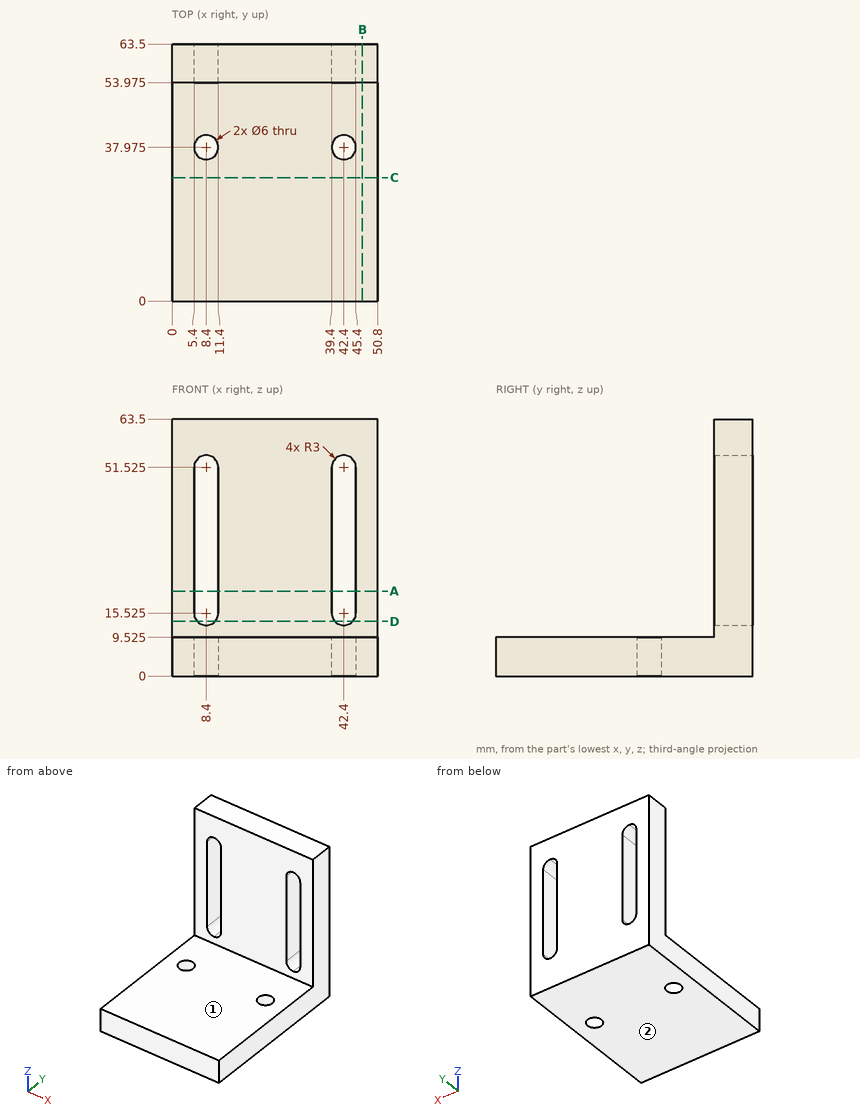
For this review, use the dimensioned drawing (mm, ordinates from the lowest corner) and the shaded views. A direction names the side the tool comes from. Give positions to 0.01 mm unless a question says otherwise; leave off trailing zeros. Write each loop counter-clockwise with the first axis right and the second up, starting at its lowest first coordinate (ties: lowest second). Pieces come first, ordered by that corner, then holes. Notation, with made-up numbers: M 7,-13 L 38,-13 A20 ccw 38,3 Z; hole C 61.25,77.25 d8. An arc over 180 degrees is marked long. Answer as a JSON object with one key per item and string values. Group by question number.
Item 1: For probe 1 along Y at (x, z) = (42.4, 6.25) (3 decimals); probe 2 along Z at (x, y) = (17, 18.5) (3 decimals); probe 3 along X at (y, z) = (55, 52), list the stretches that pass through material, from the lowest coordinate up. Write a range as [from, to].
Item 2: For pin 1 Ø9.5 at (x, y) = (8.4, 37.975) entering from +Z (3 decimals); pin 2 Ø4 at (x, y) = (28.5, 33) entering from -Z; pin 3 Ø12 at (x, z) = (43.5, 53) entering from -Y (3 decimals); pin 4 Ø12 at (y, z) = (45.5, 22.5) entering from -X, all flat-tipped, find the tip position at first contact; note any pin that passes through.
Item 3: Consider section B-B on x = 47. Write out the cut boundary in (y, z) (3 decimals).
Item 4: Consider section D-D on z = 13.5. Write out the cut boundary in (x, y) (3 decimals).
Item 5: Consider section A-A on z = 21. Write out the cut boundary in (x, y) (3 decimals).
Item 6: Tool access review of the marked faces 1 and 2: name each direction out of +Z, -Z, +X, -X, +Y, -Y from which nothing blocks a thin tool from reaching the whole face with its end or side.
Item 7: Consider section C-C on y = 30.5. Write out the cut boundary in (x, z) (3 decimals), plus the area to 3 significant figures.
Check result:
{
 "1": {"probe 1": "y = [0, 34.975], [40.975, 63.5]", "probe 2": "z = [0, 9.525]", "probe 3": "x = [0, 5.44], [11.36, 39.44], [45.36, 50.8]"},
 "2": {"pin 1": "stops at z = 9.525", "pin 2": "stops at z = 0", "pin 3": "stops at y = 53.975", "pin 4": "passes through"},
 "3": {"outline": "M 0,0 L 63.5,0 L 63.5,63.5 L 53.975,63.5 L 53.975,9.525 L 0,9.525 Z"},
 "4": {"outline": "M 0,53.975 L 6.187,53.975 L 6.187,63.5 L 0,63.5 Z; M 10.613,53.975 L 40.187,53.975 L 40.187,63.5 L 10.613,63.5 Z; M 44.613,53.975 L 50.8,53.975 L 50.8,63.5 L 44.613,63.5 Z"},
 "5": {"outline": "M 0,53.975 L 5.4,53.975 L 5.4,63.5 L 0,63.5 Z; M 11.4,53.975 L 39.4,53.975 L 39.4,63.5 L 11.4,63.5 Z; M 45.4,53.975 L 50.8,53.975 L 50.8,63.5 L 45.4,63.5 Z"},
 "6": {"face 1": "+Z, +X, -X, -Y", "face 2": "-Z, +X, -X, +Y, -Y"},
 "7": {"outline": "M 0,0 L 50.8,0 L 50.8,9.525 L 0,9.525 Z", "area": "484 mm^2"}
}
